```python
from build123d import *

# Parameters (mm, degrees)
SKETCH1_W           = 1000
SKETCH1_H           = 900
BOSS_EXTRUDE1_DEPTH = 10
SKETCH2_W           = 1000
SKETCH2_H           = 700
SKETCH2_W_2         = 980
SKETCH2_H_2         = 680
BOSS_EXTRUDE2_DEPTH = 220
SKETCH3_W           = 110
SKETCH3_H           = 170
CUT_EXTRUDE1_DEPTH  = 280
BOSS_EXTRUDE3_DEPTH = 1000


with BuildPart() as part:
    # Sketch1 → Boss-Extrude1 (new body)
    with BuildSketch(Plane(origin=(0, 0, 0), x_dir=(1, 0, 0), z_dir=(0, 1, 0))):
        Rectangle(SKETCH1_W, SKETCH1_H)
    extrude(amount=BOSS_EXTRUDE1_DEPTH)

    # Sketch2 → Boss-Extrude2 (add)
    with BuildSketch(Plane(origin=(0, 10, 0), x_dir=(1, 0, 0), z_dir=(0, 1, 0))):
        with Locations((0, 100)):
            Rectangle(SKETCH2_W, SKETCH2_H)
        with Locations((0, 100)):
            Rectangle(SKETCH2_W_2, SKETCH2_H_2, mode=Mode.SUBTRACT)
    extrude(amount=BOSS_EXTRUDE2_DEPTH)

    # Sketch3 → Cut-Extrude1 (cut)
    with BuildSketch(Plane.XY.offset(450)):
        with Locations((385, 95)):
            Rectangle(SKETCH3_W, SKETCH3_H)
    extrude(amount=-CUT_EXTRUDE1_DEPTH, mode=Mode.SUBTRACT)

    # Sketch5 → Boss-Extrude3 (add)
    with BuildSketch(Plane.ZY.offset(500)):
        Polygon((250, 230), (350, 190), (250, 190), align=None)
    extrude(amount=-BOSS_EXTRUDE3_DEPTH)


solid = part.part
```
Source: CAD feature listing. Evaluate the final solid. Frame: model axes, mm. A direction names the side the tool comes from. Give positions to 0.01 mm unless a question says otherwise; leave off trailing zeros. Order: outer loops, then holes, each group sorted by start corner. A loop starts at its lowest first (then second) coordinate and runs counter-clockwise, first axis right, second up.
(1) Section query D-D (x = 296.5). Return the cut outline in (y, z), plus the area to 3 significant figures.
(2) Section query B-B (y = 214). Return the cut outline in (x, z), plus the area to 3 significant figures.
(3) Section query C-C (z = 38.5). Return the cut outline in (x, y), plus the area to 3 significant figures.
(4) Pull-direction query (Y, two-part tool) for faces 1 (the face through (-7, 210.28, 299.3)), 2 (the face through (-500, 117, -94)), 3 (the face through (-118, 99, 250)); classes: +Y half, -Y half, draft (parallel to the pull), parting line (faces both ways), or undercut.
(5) Material intervals for line 1 along Z through (x, y) = (-350.5, 134.5); line 2 along X through (y, z) = (126, 228); line 3 along Z through (x, y) = (340, 45.5), sorted ascending.
(6) Access query for faces 4 (the face through (500, 117, -94)), 5 (the face through (490, 118, -95)), 6 (the face through (-7, 190, 301)). Directions: +Z, -Z, +X, -X, +Y, -Y. A direction counts if a zero-diameter tool reaches every point of the face in a straight line with its end or side. Return the directions, or none.
(7) Contact query for flat-ended pins moving along their axis: P1, Ø1.5, axis at x = -292.5, y = 75.5, coming from the +Z side; P2, Ø5, axis at x = -189.5, z = 25, coming from the +Y side. Output: stop coordinate, or through.
(8) Section query A-A (z = 285). Return the cut outline in (x, y), plus the area to 3 significant figures.
Outcome:
1. outline: (0, -450) - (230, -450) - (230, -440) - (10, -440) - (10, 240) - (230, 240) - (230, 250) - (190, 350) - (190, 250) - (10, 250) - (10, 450) - (0, 450) - close
1. area: 15,400 mm2
2. outline: (-500, -450) - (500, -450) - (500, 290) - (-500, 290) - close; hole (-490, -440) - (490, -440) - (490, 240) - (-490, 240) - close
2. area: 73,600 mm2
3. outline: (-500, 0) - (500, 0) - (500, 230) - (490, 230) - (490, 10) - (-490, 10) - (-490, 230) - (-500, 230) - close
3. area: 14,400 mm2
4. face 1: +Y half
4. face 2: draft
4. face 3: undercut
5. line 1: z = -450 to -440, 240 to 250
5. line 2: x = -500 to -490, 490 to 500
5. line 3: z = -450 to -440
6. face 4: +Z, -Z, +X, +Y, -Y
6. face 5: +Y
6. face 6: +Z, +X, -X
7. P1: stops at z = 250
7. P2: stops at y = 10
8. outline: (-500, 0) - (500, 0) - (500, 10) - (-500, 10) - close; (-500, 190) - (500, 190) - (500, 216) - (-500, 216) - close
8. area: 36,000 mm2
